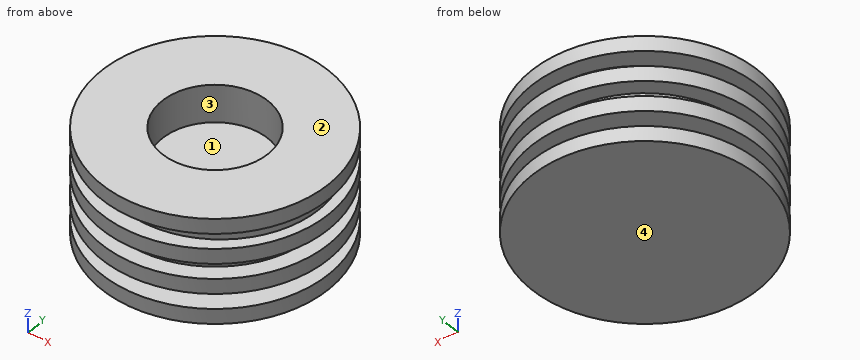
from build123d import *

# Parameters (mm, degrees)
SKETCH_1_R          = 15
EXTRUDE_1_DEPTH     = 2
SKETCH_3_R          = 12.5
EXTRUDE_2_DEPTH     = 2
SKETCH_4_R          = 15
EXTRUDE_3_DEPTH     = 2
SKETCH_5_R          = 13
EXTRUDE_4_DEPTH     = 2
SKETCH_6_R          = 15
EXTRUDE_5_DEPTH     = 2
SKETCH_7_R          = 13
EXTRUDE_6_DEPTH     = 2
SKETCH_8_R          = 15
EXTRUDE_7_DEPTH     = 2
SKETCH_9_R          = 7
CUT_EXTRUDE_1_DEPTH = 5


with BuildPart() as part:
    # 草图1 → 凸台-拉伸1 (new body)
    with BuildSketch(Plane.XY):
        Circle(SKETCH_1_R)
    extrude(amount=EXTRUDE_1_DEPTH)

    # 草图3 → 凸台-拉伸2 (add)
    with BuildSketch(Plane.XY.offset(2)):
        Circle(SKETCH_3_R)
    extrude(amount=EXTRUDE_2_DEPTH)

    # 草图4 → 凸台-拉伸3 (add)
    with BuildSketch(Plane.XY.offset(4)):
        Circle(SKETCH_4_R)
    extrude(amount=EXTRUDE_3_DEPTH)

    # 草图5 → 凸台-拉伸4 (add)
    with BuildSketch(Plane.XY.offset(6)):
        Circle(SKETCH_5_R)
    extrude(amount=EXTRUDE_4_DEPTH)

    # 草图6 → 凸台-拉伸5 (add)
    with BuildSketch(Plane.XY.offset(8)):
        Circle(SKETCH_6_R)
    extrude(amount=EXTRUDE_5_DEPTH)

    # 草图7 → 凸台-拉伸6 (add)
    with BuildSketch(Plane.XY.offset(10)):
        with Locations((0.736194689, 0)):
            Circle(SKETCH_7_R)
    extrude(amount=EXTRUDE_6_DEPTH)

    # 草图8 → 凸台-拉伸7 (add)
    with BuildSketch(Plane.XY.offset(12)):
        Circle(SKETCH_8_R)
    extrude(amount=EXTRUDE_7_DEPTH)

    # 草图9 → 切除-拉伸1 (cut)
    with BuildSketch(Plane.XY.offset(14)):
        Circle(SKETCH_9_R)
    extrude(amount=-CUT_EXTRUDE_1_DEPTH, mode=Mode.SUBTRACT)


solid = part.part
The model under review builds one solid part; all positions refer to its coordinate system, in mm. Face numbers are marked on the shaded views. A direction names the side the tool comes from. Coordinates: 2 decimals unless noted, no trailing zeros. Order: outer loops, then holes, each group sorted by start corner. A loop starts at its lowest first (then second) coordinate and runs counter-clockwise, first axis right, second up. Notation, with made-up numbers: (34, 20.5) -> (79, 20.5) arc R19 ccw to (79, 47.5) -> close; hole circle Ø2 at (19.25, 36). An arc over 180 degrees is marked (long way). Answer in a Markdown table with one row per item.
(1) Machinability: for the marked faces 1 and 2, which of the approach directions +Z, -Z, +X, -X, +Y, -Y give a long, thin tool a straight path to every point of the face, cutting with its end or side? Answer none if there is none.
Answers:
| item | result |
|---|---|
| face 1 | +Z |
| face 2 | +Z, +X, -X, +Y, -Y |
(2) Consider section D-D (z = 2.5). Write out the cut boundary in (x, y), plus the area to 3 significant figures.
Answers:
| item | result |
|---|---|
| outline | circle Ø25 at (0, 0) |
| area | 491 mm² |
(3) The part is to be moulded in two halves that separate along Y. For the marked faces 3 and 4, say which applies: +Y half, -Y half, draft (parallel to the pull), parting line (faces both ways), or undercut.
Answers:
| item | result |
|---|---|
| face 3 | undercut |
| face 4 | draft |
(4) Consider section A-A (z = 10.5). Write out the cut boundary in (x, y), plus the area to 3 significant figures.
Answers:
| item | result |
|---|---|
| outline | circle Ø26 at (0.74, 0); hole circle Ø14 at (0, 0) |
| area | 377 mm² |
(5) Wall thickness on line 1 along Z through (x, y) = (10.75, -7); line 2 along Y through (x, z) = (0, 11.85); line 3 along Z through (x, y) = (6, 2): over which ranges is each line inside the solid? List them lowest first.
Answers:
| item | result |
|---|---|
| line 1 | 0 to 2, 4 to 14 |
| line 2 | -12.98 to -7, 7 to 12.98 |
| line 3 | 0 to 9 |
(6) Insertion check: pin 1 (6 mm diameter, centred on x = -7, z = 6.5, fed in from +Y); pin 2 (2 mm diameter, centred on x = -6, z = 5, fed in from +Y); pin 3 (6 mm diameter, centred on x = 2, y = 0, fed in from +Z). Each pin has a flat end and moves straight along its axis. Give the tip position at first contact, or say it passes through.
Answers:
| item | result |
|---|---|
| pin 1 | y = 14.45 |
| pin 2 | y = 14.14 |
| pin 3 | z = 9 |
(7) Consider section C-C (x = -9.25). Write out the cut boundary in (y, z).
Answers:
| item | result |
|---|---|
| outline | (-11.81, 0) -> (11.81, 0) -> (11.81, 2) -> (8.41, 2) -> (8.41, 4) -> (11.81, 4) -> (11.81, 6) -> (9.13, 6) -> (9.13, 8) -> (11.81, 8) -> (11.81, 10) -> (8.32, 10) -> (8.32, 12) -> (11.81, 12) -> (11.81, 14) -> (-11.81, 14) -> (-11.81, 12) -> (-8.32, 12) -> (-8.32, 10) -> (-11.81, 10) -> (-11.81, 8) -> (-9.13, 8) -> (-9.13, 6) -> (-11.81, 6) -> (-11.81, 4) -> (-8.41, 4) -> (-8.41, 2) -> (-11.81, 2) -> close |
